```python
from build123d import *

# Parameters (mm, degrees)
SKETCH1_W           = 23.622
SKETCH1_H           = 22.352
BOSS_EXTRUDE1_DEPTH = 5.8674
SKETCH3_W           = 4.953
SKETCH3_H           = 1.524
BOSS_EXTRUDE2_DEPTH = 11.7348
SKETCH4_R           = 5.8674
BOSS_EXTRUDE3_DEPTH = 1.4478
SKETCH5_R           = 1.96215
BOSS_EXTRUDE4_DEPTH = 2.6162
SKETCH6_W           = 3.220759804
SKETCH6_H           = 5.4864
BOSS_EXTRUDE5_DEPTH = 1.4478


with BuildPart() as part:
    # Sketch1 → Boss-Extrude1 (new body, symmetric)
    with BuildSketch(Plane.XY):
        Rectangle(SKETCH1_W, SKETCH1_H)
    extrude(amount=BOSS_EXTRUDE1_DEPTH, both=True)

    # Sketch3 → Boss-Extrude2 (add)
    with BuildSketch(Plane.XY.offset(5.8674)):
        with Locations((-14.2875, 4.6228)):
            Rectangle(SKETCH3_W, SKETCH3_H)
        with Locations((14.2875, 4.6228)):
            Rectangle(SKETCH3_W, SKETCH3_H)
    extrude(amount=-BOSS_EXTRUDE2_DEPTH)

    # Sketch4 → Boss-Extrude3 (add)
    with BuildSketch(Plane(origin=(0, 11.176, 0), x_dir=(1, 0, 0), z_dir=(0, 1, 0))):
        with Locations((5.9436, 0)):
            Circle(SKETCH4_R)
    extrude(amount=BOSS_EXTRUDE3_DEPTH)

    # Sketch5 → Boss-Extrude4 (add)
    with BuildSketch(Plane(origin=(0, 12.6238, 0), x_dir=(1, 0, 0), z_dir=(0, 1, 0))):
        with Locations((5.9436, 0)):
            Circle(SKETCH5_R)
    extrude(amount=BOSS_EXTRUDE4_DEPTH)

    # Sketch6 → Boss-Extrude5 (add)
    with BuildSketch(Plane(origin=(0, 12.6238, 0), x_dir=(1, 0, 0), z_dir=(0, 1, 0))):
        with Locations((-0.853420098, 0)):
            Rectangle(SKETCH6_W, SKETCH6_H)
    extrude(amount=-BOSS_EXTRUDE5_DEPTH)


solid = part.part
```
Geometry check sheet. Reference: the model listing, model coordinates, mm. A direction names the side the tool comes from. Round coordinates to 2 decimals unless told otherwise and drop trailing zeros. Order: outer loops, then holes, each group sorted by start corner. A loop starts at its lowest first (then second) coordinate and runs counter-clockwise, first axis right, second up. Notation, with made-up numbers: (33, -19.5) -> (39, -19.5) arc R25 ccw to (39, 12.5) -> close; hole circle Ø4 at (4.25, 24.25). An arc over 180 degrees is marked (long way). Return JSON: item names as keys, results as strings. Group by question number.
Q1. Material ranges on probe 1 along Y at (x, z) = (-4.5, -1); probe 2 along X at (y, z) = (10.25, 4.25); probe 3 along Y at (x, z) = (15, 5.25), recorded low to high. Write a range as from..to.
Q2. Section check C-C, the plane z = -1. Record the boundary of the cut face in (x, y).
Q3. Section check D-D, the plane x = 11. Record the boundary of the cut face in (y, z).
Q4. Section check B-B, the plane y = 1.5. Record the boundary of the cut face in (x, z).
Q5. Section check A-A, the plane x = 4.5. Record the boundary of the cut face in (y, z), plus the area to 3 significant figures.
Q6. Gauge pin test, flat ends, axial feed: pin 1 (1.2 mm diameter, centred on x = -1.5, y = 11.5, fed in from -Z); pin 2 (4.5 mm diameter, centred on y = 8.5, z = -1, fed in from +X); pin 3 (3 mm diameter, centred on x = 8.5, z = -3.5, fed in from +Y); pin 4 (1.5 mm diameter, centred on x = -14.5, z = -2.5, fed in from -Y). Record the tip position at first contact, or that the pin passes through.
Q7. Tool access check on faces 1 (the flat face through (11.811, 8, 0)), 2 (the flat face through (-1, 12, -2.743)), 3 (the cylindrical face through (11.807, 11.89, 0.218)). Record the directions out of +Z, -Z, +X, -X, +Y, -Y that give a thin tool (end or side, any length) a straight path to the whole face; none if there is none.
Numbers:
{
 "1": {"probe 1": "-11.18..11.18", "probe 2": "-11.81..11.81", "probe 3": "3.86..5.38"},
 "2": {"outline": "(-16.76, 3.86) -> (-11.81, 3.86) -> (-11.81, -11.18) -> (11.81, -11.18) -> (11.81, 3.86) -> (16.76, 3.86) -> (16.76, 5.38) -> (11.81, 5.38) -> (11.81, 11.18) -> (11.73, 11.18) -> (11.73, 12.62) -> (7.63, 12.62) -> (7.63, 15.24) -> (4.26, 15.24) -> (4.26, 12.62) -> (-2.46, 12.62) -> (-2.46, 11.18) -> (-11.81, 11.18) -> (-11.81, 5.38) -> (-16.76, 5.38) -> close"},
 "3": {"outline": "(-11.18, -5.87) -> (11.18, -5.87) -> (11.18, -2.98) -> (12.62, -2.98) -> (12.62, 2.98) -> (11.18, 2.98) -> (11.18, 5.87) -> (-11.18, 5.87) -> close"},
 "4": {"outline": "(-11.81, -5.87) -> (11.81, -5.87) -> (11.81, 5.87) -> (-11.81, 5.87) -> close"},
 "5": {"outline": "(-11.18, -5.87) -> (11.18, -5.87) -> (11.18, -5.69) -> (12.62, -5.69) -> (12.62, -1.33) -> (15.24, -1.33) -> (15.24, 1.33) -> (12.62, 1.33) -> (12.62, 5.69) -> (11.18, 5.69) -> (11.18, 5.87) -> (-11.18, 5.87) -> close", "area": "286 mm^2"},
 "6": {"pin 1": "z = -5.87", "pin 2": "x = 11.81", "pin 3": "y = 12.62", "pin 4": "y = 3.86"},
 "7": {"face 1": "+Z, -Z, +X, +Y", "face 2": "-Z, -X, +Y", "face 3": "+Y"}
}
